from build123d import *

# Parameters (mm, degrees)
PAD_DEPTH    = 49
PAD001_DEPTH = 150
PAD002_DEPTH = 49
SKETCH003_R  = 2.75
PAD003_DEPTH = 3
SKETCH004_W  = 5.8
SKETCH004_H  = 3.15
POCKET_DEPTH = 49
CHAMFER_SIZE = 0.8


with BuildPart() as part:
    # Sketch → Pad (new body)
    with BuildSketch(Plane.YZ):
        Polygon((0, 0), (-19, 0), (-19, 1.5), (-15.5, 5), (-25.5, 5), (-25.5, 12.5), (0, 12.5), align=None)
        Polygon((-10.7, 6.954163), (-10.7, 5.545837), (-9.704163, 4.55), (-8.295837, 4.55), (-7.3, 5.545837), (-7.3, 6.954163), (-8.295837, 7.95), (-9.704163, 7.95), align=None, mode=Mode.SUBTRACT)
    pad = extrude(amount=PAD_DEPTH)

    # Sketch001 (on Face16 of Pad) → Pad001 (join)
    with BuildSketch(Plane(origin=(0, 0, 0), x_dir=(0, 1, 0), z_dir=(-1, 0, 0))):
        Polygon((0, 0), (0, 11.7), (-25.5, 11.7), (-25.5, -12.5), (0, -12.5), align=None)
        Polygon((-9.704163, -4.55), (-10.7, -5.545837), (-10.7, -6.954163), (-9.704163, -7.95), (-8.295837, -7.95), (-7.3, -6.954163), (-7.3, -5.545837), (-8.295837, -4.55), align=None, mode=Mode.SUBTRACT)
        Polygon((-9.704163, 7.95), (-10.7, 6.954163), (-10.7, 5.545837), (-9.704163, 4.55), (-8.295837, 4.55), (-7.3, 5.545837), (-7.3, 6.954163), (-8.295837, 7.95), align=None, mode=Mode.SUBTRACT)
    pad001 = extrude(amount=PAD001_DEPTH)

    # Sketch002 (on Face16 of Pad001) → Pad002 (join)
    with BuildSketch(Plane(origin=(-150, 0, 0), x_dir=(0, 1, 0), z_dir=(-1, 0, 0))):
        Polygon((0, 11.7), (-25.5, 11.7), (-25.5, -5), (-17.212132, -5), (-17.212132, -3.5), (-20.212132, -0.5), (-20.212132, 0), (0, 0), align=None)
        Polygon((-9.704163, 7.95), (-10.7, 6.954163), (-10.7, 5.545837), (-9.704163, 4.55), (-8.295837, 4.55), (-7.3, 5.545837), (-7.3, 6.954163), (-8.295837, 7.95), align=None, mode=Mode.SUBTRACT)
    pad002 = extrude(amount=PAD002_DEPTH)

    # Mirrored: Pad002, Pad001, Pad across Sketch002 V_Axis
    add(pad002.mirror(Plane(origin=(-150, 0, 0), x_dir=(-1, 0, 0), z_dir=(0, 1, 0))))
    add(pad001.mirror(Plane(origin=(-150, 0, 0), x_dir=(-1, 0, 0), z_dir=(0, 1, 0))))
    add(pad.mirror(Plane(origin=(-150, 0, 0), x_dir=(-1, 0, 0), z_dir=(0, 1, 0))))

    # Sketch003 (on Face30 of Mirrored) → Pad003 (join)
    with BuildSketch(Plane.YX):
        with Locations((0, 44.1)):
            Circle(SKETCH003_R)
        with Locations((0, 4.9)):
            Circle(SKETCH003_R)
    extrude(amount=PAD003_DEPTH)

    # Sketch004 (on Face8 of Pad003) → Pocket (cut)
    with BuildSketch(Plane(origin=(-199, 0, 0), x_dir=(0, 1, 0), z_dir=(-1, 0, 0))):
        with Locations((0, 1.575)):
            Rectangle(SKETCH004_W, SKETCH004_H)
    extrude(amount=-POCKET_DEPTH, mode=Mode.SUBTRACT)

    # Chamfer
    chamfer_edges = [part.edges().sort_by_distance(p)[0] for p in [
        (-50.5, -25.5, 12.5),
        (49, 0, 12.5),
        (-50.5, 25.5, 12.5),
        (-150, 0, 12.5),
        (-99.5, 25.5, -11.7),
        (-199, 25.5, -3.35),
        (-174.5, 25.5, 5),
        (-150, 25.5, 8.75),
        (49, 25.5, 8.75),
        (24.5, 25.5, 5),
        (0, 25.5, -3.35),
        (-199, -17.212132, 4.25),
        (-199, -21.356066, 5),
        (-199, -25.5, -3.35),
        (-199, 0, -11.7),
        (-199, 21.356066, 5),
        (-199, 17.212132, 4.25),
        (-199, 18.712132, 2),
        (-199, 20.212132, 0.25),
        (-199, 11.556066, 0),
        (-199, 2.9, -1.575),
        (-199, 0, -3.15),
        (-199, -2.9, -1.575),
        (-199, -11.556066, 0),
        (-199, -20.212132, 0.25),
        (-199, -18.712132, 2),
        (-199, -10.202082, -7.452082),
        (-199, -9, -7.95),
        (-199, -10.7, -6.25),
        (-199, -7.797918, -7.452082),
        (-199, -10.202082, -5.047918),
        (-199, -7.3, -6.25),
        (-199, -9, -4.55),
        (-199, -7.797918, -5.047918),
        (-199, 10.202082, -7.452082),
        (-199, 9, -7.95),
        (-199, 10.7, -6.25),
        (-199, 7.797918, -7.452082),
        (-199, 10.202082, -5.047918),
        (-199, 7.3, -6.25),
        (-199, 9, -4.55),
        (-199, 7.797918, -5.047918),
        (24.5, -25.5, 5),
        (49, -25.5, 8.75),
        (-150, -25.5, 8.75),
        (-174.5, -25.5, 5),
        (-99.5, -25.5, -11.7),
        (0, -25.5, -3.35),
        (0, 0, -11.7),
        (49, -17.25, 3.25),
        (49, -19, 0.75),
        (49, 0, 0),
        (49, 19, 0.75),
        (49, 17.25, 3.25),
        (49, 20.5, 5),
        (49, -20.5, 5),
        (49, -10.7, 6.25),
        (49, -10.202082, 7.452082),
        (49, -9, 7.95),
        (49, -7.797918, 7.452082),
        (49, -7.3, 6.25),
        (49, -7.797918, 5.047918),
        (49, -9, 4.55),
        (49, -10.202082, 5.047918),
        (49, 10.7, 6.25),
        (49, 10.202082, 5.047918),
        (49, 9, 4.55),
        (49, 7.797918, 5.047918),
        (49, 7.3, 6.25),
        (49, 7.797918, 7.452082),
        (49, 9, 7.95),
        (49, 10.202082, 7.452082),
        (44.1, -2.75, -3),
        (4.9, -2.75, -3),
    ]]
    chamfer(chamfer_edges, length=CHAMFER_SIZE)


solid = part.part
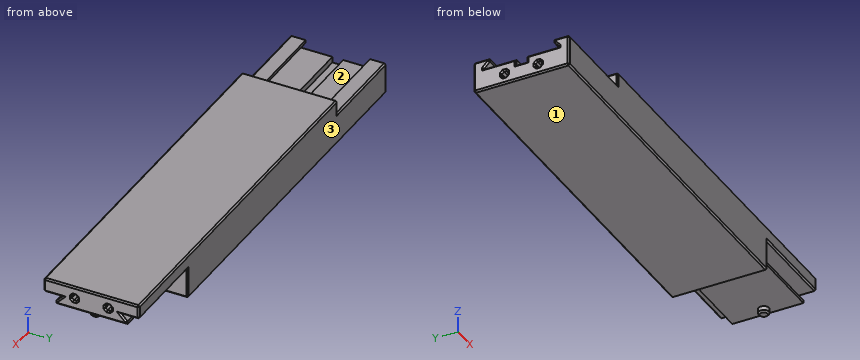
Geometry: final body of the model. Coordinates: model frame, mm. Face numbers are marked on the shaded views. Coordinates: 2 decimals unless noted, no trailing zeros. One line per question, with ' | ' between items. Start each with the question number.
Item 1: Ray query, probe 1 along Y at (x, z) = (-98, -6); probe 2 along Z at (x, y) = (4, 18.5); probe 3 along Z at (x, y) = (-122, 10.5). Return the intervals inside material, ascending. Write a range as [from, to].
Item 2: Draft query along Y for the marked faces 1, 2 and 3. Return one class per face: released by +Y, released by -Y, zero draft, split by the parting line, or undercut.
Item 3: Cut plane A-A, the plane x = -145.5. Count the separate pieces of the cut face and the enclosed holes in it, then the cut area to 3 significant figures.
Item 4: Pin query (flat end, axial travel): pin 1 Ø6 at (x, y) = (-169.5, -19) entering from +Z; pin 2 Ø7.5 at (x, y) = (34.5, 21) entering from -Z; pin 3 Ø3 at (y, z) = (2.5, -2.5) entering from +X. Return the tip coordinate at first contact, or that it passes through.
A:
1) probe 1: y = [-25.5, -10.7], [-7.3, 7.3], [10.7, 25.5] | probe 2: z = [0, 2], [5, 12.5] | probe 3: z = [-11.7, -7.15], [-5.35, 5.35], [7.15, 12.5]
2) face 1: zero draft | face 2: undercut | face 3: released by +Y
3) separate pieces: 1 | enclosed holes: 4 | area: 1,190 mm2
4) pin 1: stops at z = 5 | pin 2: stops at z = 0 | pin 3: stops at x = 46.65
